Part model, mm, in its own coordinate system. Face numbers are marked on the shaded views. A direction names the side the tool comes from. Round coordinates to 2 decimals unless told otherwise and drop trailing zeros. Loops run counter-clockwise (first coordinate to the right, second up) from the corner with the lowest first, then second, coordinate; pieces in that order, holes last. Notation, with made-up numbers: M 28.25,52 L 68.25,52 A9 ccw 68.25,63 Z; hole C -4,75.5 d7. An arc over 180 degrees is marked long. Put each result on its own line as item: value. Start each with the question number.
1) Probe line 1 along Y through (x, z) = (294.5, -3.5); line 2 along Z through (x, y) = (115.5, -3); line 3 along Z through (x, y) = (353.5, -63.5). List the from-to ranges inside material, lowest first.
2) Which spindle directions (+Z, -Z, +X, -X, +Y, -Y) get a long thin tool onto all of the face, cutting with end or side? Do the marked faces 1, 2 and 3. Say none if no direction does.
3) Slice it at A-A on y = 0. Give the cut face in (x, z), then the cut area to 3 significant figures.
4) Slice it at C-C on y = 53.5. Give the cut face in (x, z), then the cut area to 3 significant figures.
5) Drop flat-ended pins along their axis: pin 1 Ø22.5 at (y, z) = (-29, -51.5) entering from -X; pin 2 Ø3 at (x, y) = (344, 5) entering from -Z; pin 3 Ø5 at (y, z) = (-27, 24) entering from +X. Give the stop position or say it passes through.
6) Slice it at D-D on z = -61.5. Give the cut face in (x, y).
7) Slice it at B-B on z = -38. Give the cut face in (x, y).
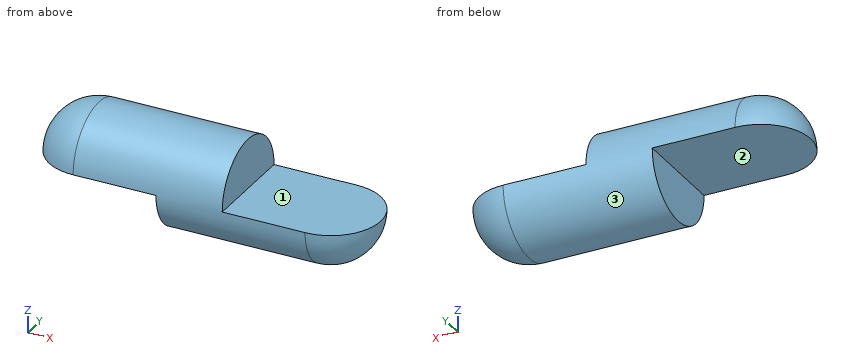
```python
from build123d import *

# Parameters (mm, degrees)
REVOLVE1_ANGLE = 180
REVOLVE2_ANGLE = 180


with BuildPart() as part:
    # Sketch1 → Revolve1 (revolve)
    with BuildSketch(Plane.XY):
        with BuildLine():
            Line((0, 75), (225, 75))
            Line((225, 75), (225, 0))
            Line((225, 0), (-75, 0))
            ThreePointArc((-75, 0), (-53.033008589, 53.033008589), (0, 75))
        make_face()
    revolve(axis=Axis((-97.796083429, 0, 0), (1, 0, 0)), revolution_arc=REVOLVE1_ANGLE)

    # Sketch1_4 → Revolve2 (revolve)
    with BuildSketch(Plane.XY):
        with BuildLine():
            Line((125, -75), (350, -75))
            ThreePointArc((350, -75), (403.033008589, -53.033008589), (425, 0))
            Line((425, 0), (125, 0))
            Line((125, 0), (125, -75))
        make_face()
    revolve(axis=Axis((-97.796083429, 0, 0), (1, 0, 0)), revolution_arc=REVOLVE2_ANGLE)


solid = part.part
```
Recorded:
1. line 1: y = -74.92 to 74.92
1. line 2: z = 0 to 74.94
1. line 3: z = -39.76 to 0
2. face 1: +Z, +X, +Y, -Y
2. face 2: -Z, -X, +Y, -Y
2. face 3: +X, -X
3. outline: M -75,0 L 125,0 L 125,-75 L 350,-75 A75 ccw 425,0 L 225,0 L 225,75 L 0,75 A75 ccw Z
3. area: 42,600 mm2
4. outline: M -52.56,0 L 125,0 L 125,-52.56 L 350,-52.56 A52.56 ccw 402.56,0 L 225,0 L 225,52.56 L 0,52.56 A52.56 ccw Z
4. area: 28,000 mm2
5. pin 1: stops at x = 125
5. pin 2: stops at z = -74.92
5. pin 3: stops at x = 225
6. outline: M 125,-42.93 L 350,-42.93 A42.93 ccw 350,42.93 L 125,42.93 Z
7. outline: M 125,-64.66 L 350,-64.66 A64.66 ccw 350,64.66 L 125,64.66 Z
